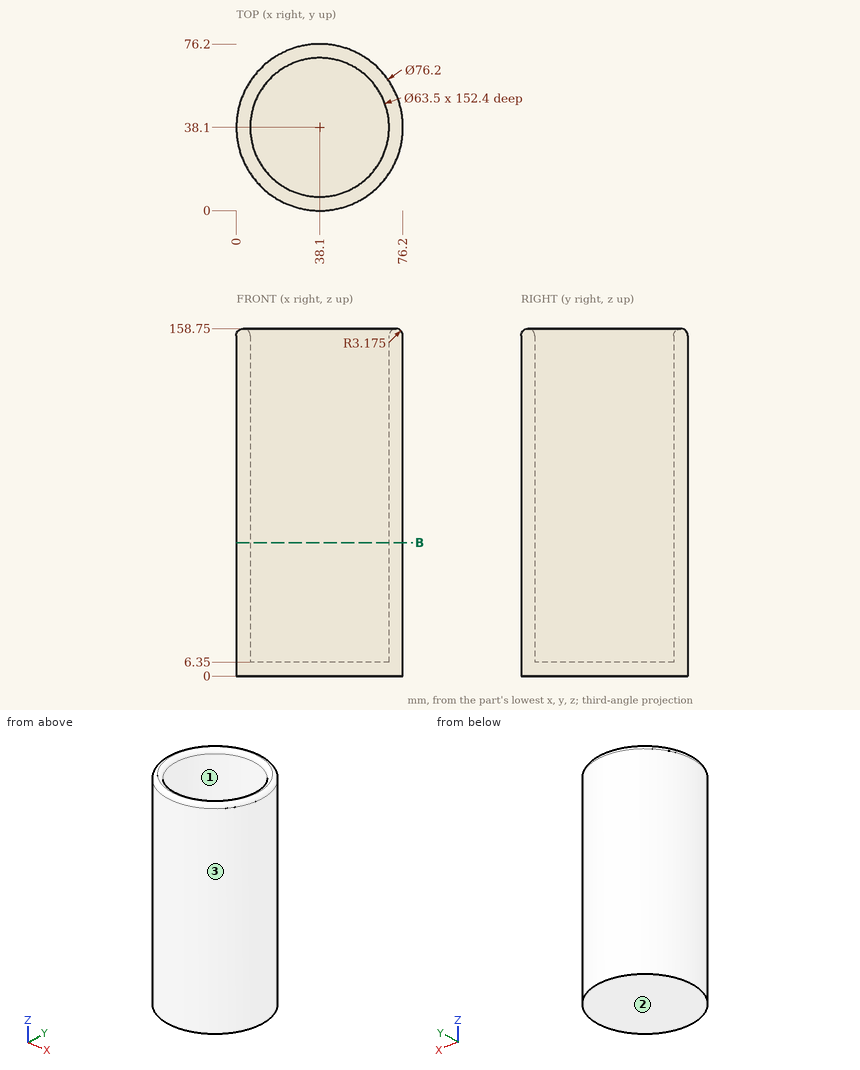
Job drawing, mm, ordinate dimensions from the low corner. One solid piece. Round coordinates to 2 decimals unless told otherwise and drop trailing zeros. Loops run counter-clockwise (first coordinate to the right, second up) from the corner with the lowest first, then second, coordinate; pieces in that order, holes last.
(1) Drop flat-ended pins along their axis: pin 1 (3 mm diameter, centred on y = 32, z = 61, fed in from +X); pin 2 (10 mm diameter, centred on x = 45.5, z = 137, fed in from -Y); pin 3 (1.5 mm diameter, centred on x = 35.5, z = 90, fed in from +Y). Give the stop position or say it passes through.
(2) Two-plate mould, pull along X, no slides. Class the marked faces 1, 2 and 3: +X half, -X half, draft (parallel to the pull), parting line (faces both ways), or undercut.
(3) Cut at B-B (z = 61). Give the cut face in (x, y), plus the area to 3 significant figures.
(4) Wall check: line 1 along Y through (x, z) = (38.1, 113.5); line 2 along Z through (x, y) = (52.5, 40); line 3 along Y through (x, z) = (22, 132). Give the ranges that are in metal, low to high.
Findings below:
1. pin 1: stops at x = 75.92
1. pin 2: stops at y = 0.08
1. pin 3: stops at y = 76.16
2. face 1: undercut
2. face 2: draft
2. face 3: parting line
3. outline: circle Ø76.2 at (38.1, 38.1); hole circle Ø63.5 at (38.1, 38.1)
3. area: 1,390 mm2
4. line 1: y = 0 to 6.35, 69.85 to 76.2
4. line 2: z = 0 to 6.35
4. line 3: y = 3.57 to 10.73, 65.47 to 72.63
